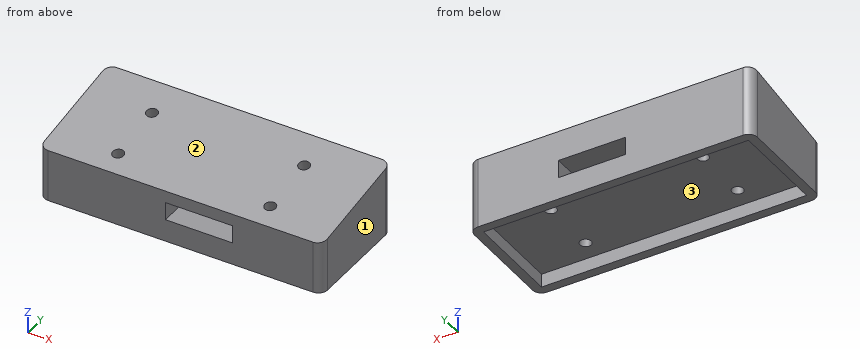
```python
from build123d import *

# Parameters (mm, degrees)
F0_W      = 63.25
F0_H      = 25.5
F0_W_2    = 59.25
F0_H_2    = 21.5
F1_DEPTH  = 20
F3_DEPTH  = 3
F4_DEPTH  = 64
F5_W      = 15
F5_H      = 4
F6_DEPTH  = 30
F8_DEPTH  = 70
F9_R      = 2
F10_R     = 1.25
F11_DEPTH = 25


with BuildPart() as f1:
    # F0 (on Top) → F1 (new body)
    with BuildSketch(Plane.XY):
        Rectangle(F0_W, F0_H)
        Rectangle(F0_W_2, F0_H_2, mode=Mode.SUBTRACT)
        Rectangle(F0_W_2, F0_H_2)
    extrude(amount=F1_DEPTH)

    # F0 (on Top) → F3 (cut)
    with BuildSketch(Plane.XY):
        Rectangle(F0_W_2, F0_H_2)
    extrude(amount=F3_DEPTH, mode=Mode.SUBTRACT)

    # F2 (on face) → F4 (cut)
    with BuildSketch(Plane.YZ.offset(31.625)):
        Polygon((-12.75, 15.9456129), (12.75, 20), (-12.75, 20), align=None)
    extrude(amount=-F4_DEPTH, mode=Mode.SUBTRACT)

    # F5 (on face) → F6 (cut)
    with BuildSketch(Plane.XZ.offset(12.75)):
        with Locations((4.125, 7)):
            Rectangle(F5_W, F5_H)
    extrude(amount=-F6_DEPTH, mode=Mode.SUBTRACT)

    # F7 (on face) → F8 (cut)
    with BuildSketch(Plane.YZ.offset(31.625)):
        Polygon((-12.75, 11.6711445153), (12.75, 15.7628711313), (12.75, 20), (-12.75, 15.9456129), align=None)
    extrude(amount=-F8_DEPTH, mode=Mode.SUBTRACT)

    # F9
    f9_edges = [f1.edges().sort_by_distance(p)[0] for p in [
        (-31.625, 12.75, 7.881436),
        (31.625, 12.75, 7.881436),
        (-31.625, -12.75, 5.835572),
        (31.625, -12.75, 5.835572),
    ]]
    fillet(f9_edges, radius=F9_R)

    # F10 (on face) → F11 (cut)
    with BuildSketch(Plane(origin=(0, -2.1457810388, 13.3726960826), x_dir=(1, 0, 0), z_dir=(0, -0.1584332105, 0.9873696966))):
        with Locations((-17, 7.0863259119)):
            Circle(F10_R)
        with Locations((-17, -5.6142242387)):
            Circle(F10_R)
        with Locations((17, 7.0863259119)):
            Circle(F10_R)
        with Locations((17, -5.6142242387)):
            Circle(F10_R)
    extrude(amount=-F11_DEPTH, mode=Mode.SUBTRACT)


solid = f1.part
```
Input: part model. Units: mm. Frame: model coordinates. Face numbers are marked on the shaded views. Round coordinates to 2 decimals unless told otherwise and drop trailing zeros. Loops run counter-clockwise (first coordinate to the right, second up) from the corner with the lowest first, then second, coordinate; pieces in that order, holes last. Notation, with made-up numbers: (16, 29) - (21, 29) arc R25 cw to (21, 43) - close; hole circle Ø5 at (-27.5, -2.75). An arc over 180 degrees is marked (long way). One line per item, written item: value. Start each with the question number.
(1) Section D-D, the plane x = 22. Return loops of the section in (y, z).
(2) Section A-A, the plane z = 1.5. Return loops of the section in (x, y) (3 decimals), plus the area to 3 significant figures.
(3) Ray query, line 1 (X direction, y = 9, z = 1.5) (3 decimals); line 2 (Y direction, x = -8, z = 2); line 3 (X direction, y = 8.75, z = 7.75) (3 decimals). Return the intervals inside material, ascending. Write a range as [from, to].
(4) Section B-B, the plane x = 7. Return loops of the section in (y, z), plus the area to 3 significant figures.
(5) Section C-C, the plane y = 0. Return loops of the section in (x, z) (3 decimals), plus the area to 3 significant figures.
(6) Contact query for flat-ended pins moving along their axis: P1, Ø6, axis at x = -3, y = 0, coming from the +Z side; P2, Ø4.5, axis at x = 2, y = -3, coming from the +Z side; P3, Ø7.5, axis at x = 6, y = 4.5, coming from the -Z side. Output: stop coordinate, or through.
(7) Draft query along Y for the marked faces 1, 2 and 3. Return one class per face: +Y half, -Y half, draft (parallel to the pull), parting line (faces both ways), or undercut.
Results below:
1. outline: (-12.75, 0) - (-10.75, 0) - (-10.75, 3) - (10.75, 3) - (10.75, 0) - (12.75, 0) - (12.75, 15.76) - (-12.75, 11.67) - close
2. outline: (-31.625, -10.75) arc R2 ccw to (-29.625, -12.75) - (29.625, -12.75) arc R2 ccw to (31.625, -10.75) - (31.625, 10.75) arc R2 ccw to (29.625, 12.75) - (-29.625, 12.75) arc R2 ccw to (-31.625, 10.75) - close; hole (-29.625, -10.75) - (29.625, -10.75) - (29.625, 10.75) - (-29.625, 10.75) - close
2. area: 336 mm^2
3. line 1: [-31.625, -29.625], [29.625, 31.625]
3. line 2: [-12.75, -10.75], [10.75, 12.75]
3. line 3: [-31.625, -3.375], [11.625, 31.625]
4. outline: (-12.75, 0) - (-10.75, 0) - (-10.75, 3) - (10.75, 3) - (10.75, 0) - (12.75, 0) - (12.75, 5) - (-12.75, 5) - close; (-12.75, 9) - (12.75, 9) - (12.75, 15.76) - (-12.75, 11.67) - close
4. area: 183 mm^2
5. outline: (-31.625, 0) - (-29.625, 0) - (-29.625, 3) - (29.625, 3) - (29.625, 0) - (31.625, 0) - (31.625, 13.717) - (-31.625, 13.717) - close; hole (-3.375, 5) - (11.625, 5) - (11.625, 9) - (-3.375, 9) - close
5. area: 630 mm^2
6. P1: z = 14.2
6. P2: z = 13.6
6. P3: z = 3
7. face 1: draft
7. face 2: -Y half
7. face 3: undercut
